Design review of the part built by this model. Coordinates are the model's own, in mm. A direction names the side the tool comes from. Round coordinates to 2 decimals unless told otherwise and drop trailing zeros. Loops run counter-clockwise (first coordinate to the right, second up) from the corner with the lowest first, then second, coordinate; pieces in that order, holes last. Notation, with made-up numbers: M 26.25,-39 L 53.25,-39 A24 cw 53.25,-9 Z; hole C -14,13.5 d4. An arc over 180 degrees is marked long. One line per item, written item: value. Start each with the question number.
Item 1: For line 1 along Y through (x, z) = (73, -4.2); line 2 along X through (y, z) = (-15, -2.55); line 3 along Y through (x, z) = (52.5, -4.1), list the stretches that pass through material, from the lowest coordinate up.
Item 2: We need section A-A (z = -1.75). Write out the cut boundary in (x, y).
Item 3: For faces 1 (the flat face through (123, -23.539, -2)), 2 (the flat face through (-63.302, -27, -2)), 3 (the flat face through (119.698, 26, -2)), 4 (the flat face through (-63.302, 26, -2)), list the 3-axis set-ups (+Z, -Z, +X, -X, +Y, -Y) from which the entire face can be reached by the end or side of a thin tool; tool diameter is ignored.
Item 4: We need section B-B (x = -45.5). Write out the cut boundary in (y, z).
Item 5: Mouldability with a two-part tool opening along X and no side actions: class faces 5 (the flat face through (-67, 22.461, -2)), 6 (the flat face through (30, 0, -3)), 7 (the flat face through (126.698, 0, -2)) as released by +X, released by -X, zero draft, split by the parting line, or undercut.
Item 6: Clearance check with flat-ended pins moving along their axes: pin 1 (1.5 mm diameter, centred on x = 125, z = -3.5, fed in from +Y); pin 2 (12 mm diameter, centred on x = 60, y = 19.5, fed in from +Z); pin 3 (1.5 mm diameter, centred on y = -24.5, z = -1, fed in from +X); pin 4 (2.5 mm diameter, centred on x = -63.5, z = -1.5, fed in from -Y). State where each tip first meets the part, or that it passes through.
from build123d import *

# Parameters (mm, degrees)
PAD_DEPTH       = 5
POCKET003_DEPTH = 3
SKETCH011_R     = 1.5
POCKET004_DEPTH = 10


with BuildPart() as part:
    # Sketch009 (on Face5 of Pad002) → Pad (new body)
    with BuildSketch(Plane(origin=(0, 0, 0), x_dir=(1, 0, 0), z_dir=(0, 0, -1))):
        Polygon((-63.30204, 23.538714), (-70.30204, 23.538714), (-70.30204, -22.461286), (-63.30204, -22.461286), (-63.30204, -29.461286), (119.69796, -29.461286), (119.69796, -22.461286), (126.69796, -22.461286), (126.69796, 23.538714), (119.69796, 23.538714), (119.69796, 30.538714), (-63.30204, 30.538714), align=None)
    extrude(amount=PAD_DEPTH)

    # Sketch010 (on Face13 of Pad) → Pocket003 (cut)
    with BuildSketch(Plane.XY):
        Polygon((-60.80204, -28.038714), (-60.80204, -21.038714), (-67.80204, -21.038714), (-67.80204, 19.961286), (-60.80204, 19.961286), (-60.80204, 26.961286), (117.19796, 26.961286), (117.19796, 19.961286), (124.19796, 19.961286), (124.19796, -21.038714), (117.19796, -21.038714), (117.19796, -28.038714), align=None)
    extrude(amount=-POCKET003_DEPTH, mode=Mode.SUBTRACT)

    # Sketch011 (on Face27 of Pocket003) → Pocket004 (cut)
    with BuildSketch(Plane.XY.offset(-3)):
        with Locations((-48.657681, 23.169219)):
            Circle(SKETCH011_R)
        with Locations((-34.114651, 7.669219)):
            Circle(SKETCH011_R)
        with Locations((26.342319, 22.86806)):
            Circle(SKETCH011_R)
        with Locations((-25.157681, -20.330781)):
            Circle(SKETCH011_R)
        with Locations((-56.157681, -25.330781)):
            Circle(SKETCH011_R)
        with Locations((26.342319, -25.63194)):
            Circle(SKETCH011_R)
        with Locations((52.5, -11.63194)):
            Circle(SKETCH011_R)
        with Locations((52.5, -16.63194)):
            Circle(SKETCH011_R)
        with Locations((73, 18.059744)):
            Circle(SKETCH011_R)
        with Locations((73, -20.940256)):
            Circle(SKETCH011_R)
    extrude(amount=-POCKET004_DEPTH, mode=Mode.SUBTRACT)


solid = part.part
A:
1. line 1: -30.54 to -22.44, -19.44 to 16.56, 19.56 to 29.46
1. line 2: -70.3 to -67.8, 124.2 to 126.7
1. line 3: -30.54 to -18.13, -15.13 to -13.13, -10.13 to 29.46
2. outline: M -70.3,-23.54 L -63.3,-23.54 L -63.3,-30.54 L 119.7,-30.54 L 119.7,-23.54 L 126.7,-23.54 L 126.7,22.46 L 119.7,22.46 L 119.7,29.46 L -63.3,29.46 L -63.3,22.46 L -70.3,22.46 Z; hole M -67.8,-21.04 L -60.8,-21.04 L -60.8,-28.04 L 117.2,-28.04 L 117.2,-21.04 L 124.2,-21.04 L 124.2,19.96 L 117.2,19.96 L 117.2,26.96 L -60.8,26.96 L -60.8,19.96 L -67.8,19.96 Z
3. face 1: +Z, -Z, +X, -Y
3. face 2: +Z, -Z, -X, -Y
3. face 3: +Z, -Z, +X, +Y
3. face 4: +Z, -Z, -X, +Y
4. outline: M -30.54,-5 L 29.46,-5 L 29.46,0 L 26.96,0 L 26.96,-3 L -28.04,-3 L -28.04,0 L -30.54,0 Z
5. face 5: zero draft
5. face 6: undercut
5. face 7: released by +X
6. pin 1: y = 22.46
6. pin 2: z = -3
6. pin 3: x = 119.7
6. pin 4: y = -30.54
